Here's the drawing with two shaded views (mm, measured from the low corner). I have some questions. Give positions to 0.01 mm unless a question says otherwise; leave off trailing zeros. Write each loop counter-clockwise with the first axis right and the second up, starting at its lowest first coordinate (ties: lowest second). Pieces come first, ordered by that corner, then holes. Notation, with made-up numbers: (73, -3) - (119, -3) arc R16 ccw to (119, 16) - close; hole circle Ø9 at (83, 59.25). An arc over 180 degrees is marked (long way). Answer as a JSON object with one key per item and string values. Group by question number.
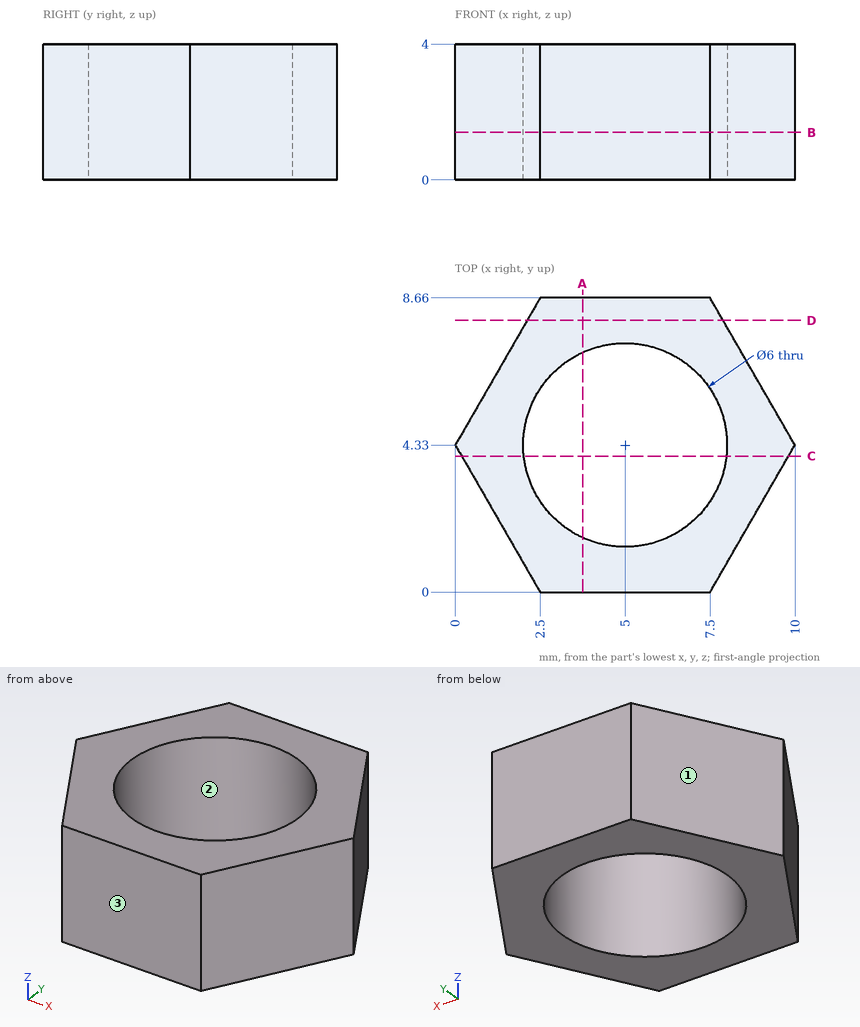
(1) I need wall thicknesses on L1, parallel to Y at x = 5, z = 1.35; L2, parallel to Y at x = 5.75, z = 0.4 (1 decimal); L3, parallel to X at y = 4, z = 1.2. Which ranges of each line are inside material? Lowest first, please.
(2) I want a section at C-C, the plane y = 4. Please give me the cut outline in (x, z).
(3) I want a section at B-B, the plane z = 1.4. Please give me the cut outline in (x, y).
(4) If we mould it in two halves opening along X, with no side actions, what happens to the marked faces 1, 2 and 3? For each: +X half, -X half, draft (parallel to the pull), parting line (faces both ways), or undercut.
(5) I want a section at A-A, the plane x = 3.75. Please give me the cut outline in (y, z), and give its area (3 significant figures).
(6) I want a section at D-D, the plane y = 8. Please give me the cut outline in (x, z).
Entries:
{
 "1": {"L1": "0 to 1.33, 7.33 to 8.66", "L2": "0 to 1.4, 7.2 to 8.7", "L3": "0.19 to 2.02, 7.98 to 9.81"},
 "2": {"outline": "(0.19, 0) - (2.02, 0) - (2.02, 4) - (0.19, 4) - close; (7.98, 0) - (9.81, 0) - (9.81, 4) - (7.98, 4) - close"},
 "3": {"outline": "(0, 4.33) - (2.5, 0) - (7.5, 0) - (10, 4.33) - (7.5, 8.66) - (2.5, 8.66) - close; hole circle Ø6 at (5, 4.33)"},
 "4": {"face 1": "-X half", "face 2": "undercut", "face 3": "draft"},
 "5": {"outline": "(0, 0) - (1.6, 0) - (1.6, 4) - (0, 4) - close; (7.06, 0) - (8.66, 0) - (8.66, 4) - (7.06, 4) - close", "area": "12.8 mm^2"},
 "6": {"outline": "(2.12, 0) - (7.88, 0) - (7.88, 4) - (2.12, 4) - close"}
}
